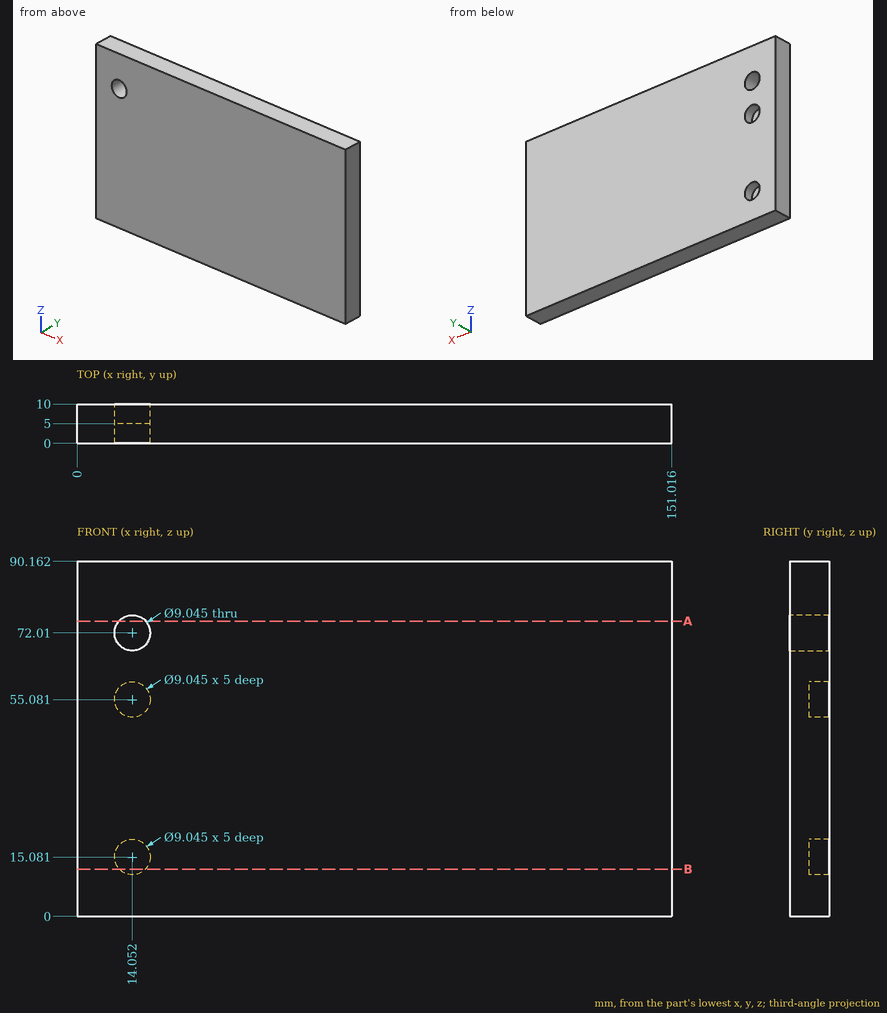
Verification items for this drawing (mm, ordinates from the low corner). Round coordinates to 2 decimals unless told otherwise and drop trailing zeros. Write each loop counter-clockwise with the first axis right and the second up, starting at its lowest first coordinate (ties: lowest second). Pieces come first, ordered by that corner, then holes. Notation, with made-up numbers: M -34,-28 L -10,-28 A26 cw -10,5 Z; hole C -36.75,-19 d3. An arc over 180 degrees is marked long. Write item = value, one per line. Start each with the question number.
1. Gauge pin test, flat ends, axial feed: pin 1 (8 mm diameter, centred on x = 14.05, z = 72.01, fed in from -Y); pin 2 (5.5 mm diameter, centred on x = 14.05, z = 15.08, fed in from +Y). Record the tip position at first contact, or that the pin passes through.
2. Section check B-B, the plane z = 12. Record the cut outline in (x, y) (1 decimal), then the cut area to 3 significant figures.
3. Section check A-A, the plane z = 75. Record the cut outline in (x, y) (1 decimal), then the cut area to 3 significant figures.
4. Scan lines: line 1 (Z direction, x = 16, y = 5.75); line 2 (X direction, y = 4.5, z = 68) (1 decimal); line 3 (X direction, y = 1.5, z = 69) (1 decimal). Record each from-to range of solid material in increasing order. Write a range as [from, to].
Results found:
q1.pin_1 = through
q1.pin_2 = 5
q2.outline = M 0,0 L 151,0 L 151,10 L 17.4,10 L 17.4,5 L 10.7,5 L 10.7,10 L 0,10 Z
q2.area = 1,480 mm^2
q3.outline = M 0,0 L 10.7,0 L 10.7,10 L 0,10 Z; M 17.4,0 L 151,0 L 151,10 L 17.4,10 Z
q3.area = 1,440 mm^2
q4.line_1 = [0, 11], [19.16, 51], [59.16, 67.93], [76.09, 90.16]
q4.line_2 = [0, 12], [16.1, 151]
q4.line_3 = [0, 10.7], [17.4, 151]
